Autodesk Inventor part; units mm, degrees
ref_plane "YZ Plane" through (0, 0, 0) normal (1, 0, 0) x (0, 1, 0)
ref_plane "XZ Plane" through (0, 0, 0) normal (0, 1, 0) x (-1, 0, 0)
ref_plane "XY Plane" through (0, 0, 0) normal (0, 0, 1) x (1, 0, 0)
sketch "Esquisse1" plane through (0, 0, 0) normal (0, 1, 0) x (-1, 0, 0)
  line L0 (60, -42) -> (60, 42)
  line L1 (55, 39) -> (57, 39)
  arc A0 (52, 42) -> (55, 39) centre (55, 42) ccw
  line L2 (52, 44) -> (52, 42)
  line L3 (55, 46) -> (-55, 46)
  circle A1 centre (55, 42.115) radius 2
  arc A2 (60, 42) -> (55, 47) centre (55, 42) ccw
  line L4 (55, 47) -> (-55, 47)
  line L5 (-55, 47) -> (55, 47)
  line L6 (51, 45) -> (-51, 45)
  line L7 (-52, 42) -> (-51, 42)
  arc A3 (-57, 39) -> (-58, 38) centre (-57, 38) ccw
  circle A4 centre (-55, 42.115) radius 2
  line L8 (-55, 39) -> (-55, 38)
  line L9 (-52, 44) -> (-52, 42)
  arc A5 (-51, 45) -> (-52, 44) centre (-51, 44) ccw
  line L10 (-55, 39) -> (-57, 39)
  arc A6 (-55, 39) -> (-52, 42) centre (-55, 42) ccw
  arc A7 (-57, 39) -> (-58, 38) centre (-57, 38) ccw
  circle A8 centre (55, -42.115) radius 2
  line L11 (-55, -39) -> (-57, -39)
  arc A9 (-52, -42) -> (-55, -39) centre (-55, -42) ccw
  line L12 (-52, -44) -> (-52, -42)
  line L13 (52, -42) -> (52, -44)
  circle A10 centre (-55, -42.115) radius 2
  line L14 (-51, -45) -> (51, -45)
  line L15 (51, -45) -> (-51, -45)
  line L16 (-55, -46) -> (55, -46)
  line L17 (-55, -47) -> (55, -47)
  line L18 (55, -47) -> (-55, -47)
  arc A11 (-51, 45) -> (-52, 44) centre (-51, 44) ccw
  line L19 (-52, 42) -> (-52, 44)
  arc A12 (-55, 46) -> (-59, 42) centre (-55, 42) ccw
  line L20 (-51, 42) -> (-51, 45)
  arc A13 (-55, 47) -> (-60, 42) centre (-55, 42) ccw
  circle A14 centre (-55, 42.115) radius 2
  line L21 (-55, 46) -> (-55, 47)
  arc A15 (-55, 47) -> (-60, 42) centre (-55, 42) ccw
  line L22 (52, -42) -> (51, -42)
  arc A16 (51, -45) -> (52, -44) centre (51, -44) ccw
  line L23 (-51, 45) -> (51, 45)
  arc A17 (52, 42) -> (55, 39) centre (55, 42) ccw
  line L24 (55, -39) -> (55, -38)
  line L25 (57, -39) -> (55, -39)
  line L26 (55, -39) -> (57, -39)
  arc A18 (55, -39) -> (52, -42) centre (55, -42) ccw
  arc A19 (57, -39) -> (58, -38) centre (57, -38) ccw
  line L27 (52, -44) -> (52, -42)
  arc A20 (51, -45) -> (52, -44) centre (51, -44) ccw
  circle A21 centre (55, -42.115) radius 2
  arc A22 (57, -39) -> (58, -38) centre (57, -38) ccw
  line L28 (58, 38) -> (58, -38)
  circle A23 centre (55, 42.115) radius 2
  line L29 (52, 42) -> (52, 44)
  line L30 (52, 42) -> (51, 42)
  arc A24 (52, 44) -> (51, 45) centre (51, 44) ccw
  line L31 (55, 39) -> (55, 38)
  arc A25 (52, 44) -> (51, 45) centre (51, 44) ccw
  arc A26 (58, 38) -> (57, 39) centre (57, 38) ccw
  arc A27 (58, 38) -> (57, 39) centre (57, 38) ccw
  line L32 (57, 39) -> (55, 39)
  line L33 (58, -38) -> (58, 38)
  line L34 (58, -38) -> (55, -38)
  line L35 (55, 46) -> (55, 47)
  arc A28 (59, 42) -> (55, 46) centre (55, 42) ccw
  arc A29 (60, 42) -> (55, 47) centre (55, 42) ccw
  line L36 (59, -42) -> (59, 42)
  line L37 (59, 42) -> (60, 42)
  line L38 (60, 42) -> (60, -42)
  line L39 (51, 45) -> (51, 42)
  arc A30 (51, 42) -> (55, 38) centre (55, 42) ccw
  line L40 (55, 38) -> (58, 38)
  arc A31 (55, -39) -> (52, -42) centre (55, -42) ccw
  arc A32 (55, -47) -> (60, -42) centre (55, -42) ccw
  line L41 (-55, -38) -> (-58, -38)
  arc A33 (-51, -42) -> (-55, -38) centre (-55, -42) ccw
  line L42 (-52, -42) -> (-51, -42)
  line L43 (-52, -42) -> (-52, -44)
  line L44 (-51, -45) -> (-51, -42)
  arc A34 (-52, -44) -> (-51, -45) centre (-51, -44) ccw
  circle A35 centre (-55, -42.115) radius 2
  line L45 (-55, -46) -> (-55, -47)
  arc A36 (-59, -42) -> (-55, -46) centre (-55, -42) ccw
  arc A37 (-60, -42) -> (-55, -47) centre (-55, -42) ccw
  line L46 (-60, -42) -> (-59, -42)
  arc A38 (-60, -42) -> (-55, -47) centre (-55, -42) ccw
  arc A39 (-58, -38) -> (-57, -39) centre (-57, -38) ccw
  line L47 (-57, 39) -> (-55, 39)
  arc A40 (-55, 39) -> (-52, 42) centre (-55, 42) ccw
  line L48 (-55, -39) -> (-55, -38)
  line L49 (-58, -38) -> (-58, 38)
  arc A41 (-52, -44) -> (-51, -45) centre (-51, -44) ccw
  arc A42 (-58, -38) -> (-57, -39) centre (-57, -38) ccw
  line L50 (-60, 42) -> (-60, -42)
  arc A43 (-52, -42) -> (-55, -39) centre (-55, -42) ccw
  line L51 (-57, -39) -> (-55, -39)
  line L52 (-58, 38) -> (-58, -38)
  line L53 (-58, 38) -> (-55, 38)
  arc A44 (-55, 38) -> (-51, 42) centre (-55, 42) ccw
  line L54 (-59, 42) -> (-60, 42)
  line L55 (-60, -42) -> (-60, 42)
  line L56 (-59, 42) -> (-59, -42)
  line L57 (55, -46) -> (55, -47)
  arc A45 (55, -38) -> (51, -42) centre (55, -42) ccw
  line L58 (51, -42) -> (51, -45)
  arc A46 (55, -46) -> (59, -42) centre (55, -42) ccw
  line L59 (59, -42) -> (60, -42)
  arc A47 (55, -47) -> (60, -42) centre (55, -42) ccw
  line L60 (-37.5, -35) -> (-22.5, -35)
  line L61 (-37.5, -35) -> (-22.5, -35)
  line L62 (-33.25, 35) -> (-37.5, 35)
  line L63 (-33.25, 35) -> (-31.25, 35)
  line L64 (-31.25, 32) -> (-33.25, 32)
  line L65 (-31.25, 35) -> (-31.25, 32)
  line L66 (-31.25, 32) -> (-33.25, 32)
  line L67 (-28.75, 35) -> (-31.25, 35)
  line L68 (-28.75, 32) -> (-28.75, 35)
  line L69 (-28.75, 32) -> (-28.75, 35)
  line L70 (-26.75, 32) -> (-28.75, 32)
  line L71 (-26.75, 32) -> (-28.75, 32)
  line L72 (-22.5, 35) -> (-37.5, 35)
  line L73 (-22.5, 35) -> (-26.75, 35)
  line L74 (-37.5, 35) -> (-37.5, -35)
  line L75 (-37.5, 35) -> (-37.5, -35)
  line L76 (-22.5, -35) -> (-22.5, 35)
  line L77 (-22.5, -35) -> (-22.5, 35)
  line L78 (-28.75, 35) -> (-26.75, 35)
  line L79 (-31.25, 35) -> (-31.25, 32)
  line L80 (-26.75, 35) -> (-26.75, 32)
  line L81 (-26.75, 35) -> (-26.75, 32)
  line L82 (-33.25, 32) -> (-33.25, 35)
  line L83 (-33.25, 32) -> (-33.25, 35)
  line L84 (-7.5, -35) -> (7.5, -35)
  line L85 (-7.5, -35) -> (7.5, -35)
  line L86 (-3.25, 35) -> (-7.5, 35)
  line L87 (-3.25, 35) -> (-1.25, 35)
  line L88 (-1.25, 32) -> (-3.25, 32)
  line L89 (-1.25, 35) -> (-1.25, 32)
  line L90 (-1.25, 32) -> (-3.25, 32)
  line L91 (1.25, 35) -> (-1.25, 35)
  line L92 (1.25, 32) -> (1.25, 35)
  line L93 (1.25, 32) -> (1.25, 35)
  line L94 (3.25, 32) -> (1.25, 32)
  line L95 (3.25, 32) -> (1.25, 32)
  line L96 (7.5, 35) -> (-7.5, 35)
  line L97 (7.5, 35) -> (3.25, 35)
  line L98 (-7.5, 35) -> (-7.5, -35)
  line L99 (-7.5, 35) -> (-7.5, -35)
  line L100 (7.5, -35) -> (7.5, 35)
  line L101 (7.5, -35) -> (7.5, 35)
  line L102 (1.25, 35) -> (3.25, 35)
  line L103 (-1.25, 35) -> (-1.25, 32)
  line L104 (3.25, 35) -> (3.25, 32)
  line L105 (3.25, 35) -> (3.25, 32)
  line L106 (-3.25, 32) -> (-3.25, 35)
  line L107 (-3.25, 32) -> (-3.25, 35)
  line L108 (22.5, -35) -> (37.5, -35)
  line L109 (22.5, -35) -> (37.5, -35)
  line L110 (26.75, 35) -> (22.5, 35)
  line L111 (26.75, 35) -> (28.75, 35)
  line L112 (28.75, 32) -> (26.75, 32)
  line L113 (28.75, 35) -> (28.75, 32)
  line L114 (28.75, 32) -> (26.75, 32)
  line L115 (31.25, 35) -> (28.75, 35)
  line L116 (31.25, 32) -> (31.25, 35)
  line L117 (31.25, 32) -> (31.25, 35)
  line L118 (33.25, 32) -> (31.25, 32)
  line L119 (33.25, 32) -> (31.25, 32)
  line L120 (37.5, 35) -> (22.5, 35)
  line L121 (37.5, 35) -> (33.25, 35)
  line L122 (22.5, 35) -> (22.5, -35)
  line L123 (22.5, 35) -> (22.5, -35)
  line L124 (37.5, -35) -> (37.5, 35)
  line L125 (37.5, -35) -> (37.5, 35)
  line L126 (31.25, 35) -> (33.25, 35)
  line L127 (28.75, 35) -> (28.75, 32)
  line L128 (33.25, 35) -> (33.25, 32)
  line L129 (33.25, 35) -> (33.25, 32)
  line L130 (26.75, 32) -> (26.75, 35)
  line L131 (26.75, 32) -> (26.75, 35)
  line L132 (55, -42) -> (-55, 42) construction
  line L133 (55, 42) -> (-55, -42) construction
  line L134 (58, -30.8976) -> (-58, -30.8976)
  point P0 (0, 0)
  point P1 (0, 0)
  point P2 (37.5, -30.8976)
  point P3 (22.5, -30.8976)
  point P4 (7.5, -30.8976)
  point P5 (-7.5, -30.8976)
  point P6 (-22.5, -30.8976)
  point P7 (-37.5, -30.8976)
  point P8 (-58, -30.8976)
extrude "Extrusion1" add sketch "Esquisse1" along normal blind 5 contours L28 L34 A45 L58 L14 L44 A33 L41 L49 L134 L74 L60 L76 L98 L84 L100 L122 L108 L124
sketch "Esquisse2" plane through (0, 5, 0) normal (0, 1, 0) x (1, 0, 0)
  line L0 (-58, 38) -> (-58, 30.8976)
  line L1 (-58, 30.8976) -> (-37.5, 30.8976)
  line L2 (-37.5, 30.8976) -> (-37.5, 35)
  line L3 (-37.5, 35) -> (-22.5, 35)
  line L4 (-22.5, 35) -> (-22.5, 30.8976)
  line L5 (-22.5, 30.8976) -> (-7.5, 30.8976)
  line L6 (-7.5, 30.8976) -> (-7.5, 35)
  line L7 (-7.5, 35) -> (7.5, 35)
  line L8 (7.5, 35) -> (7.5, 30.8976)
  line L9 (7.5, 30.8976) -> (22.5, 30.8976)
  line L10 (22.5, 30.8976) -> (22.5, 35)
  line L11 (22.5, 35) -> (37.5, 35)
  line L12 (37.5, 35) -> (37.5, 30.8976)
  line L13 (37.5, 30.8976) -> (58, 30.8976)
  line L14 (58, 30.8976) -> (58, 38)
  line L15 (58, 38) -> (55, 38)
  arc A0 (51, 42) -> (55, 38) centre (55, 42) ccw
  line L16 (51, 42) -> (51, 45)
  line L17 (51, 45) -> (-51, 45)
  line L18 (-51, 45) -> (-51, 42)
  arc A1 (-55, 38) -> (-51, 42) centre (-55, 42) ccw
  line L19 (-55, 38) -> (-58, 38)
  line L20 (-50.9, 44.9) -> (50.9, 44.9)
  line L21 (50.9, 44.9) -> (50.9, 42)
  arc A2 (50.9, 42) -> (55, 37.9) centre (55, 42) ccw
  line L22 (55, 37.9) -> (57.9, 37.9)
  line L23 (57.9, 37.9) -> (57.9, 30.9976)
  line L24 (57.9, 30.9976) -> (37.6, 30.9976)
  line L25 (37.6, 30.9976) -> (37.6, 35.1)
  line L26 (37.6, 35.1) -> (22.4, 35.1)
  line L27 (22.4, 35.1) -> (22.4, 30.9976)
  line L28 (22.4, 30.9976) -> (7.6, 30.9976)
  line L29 (7.6, 30.9976) -> (7.6, 35.1)
  line L30 (7.6, 35.1) -> (-7.6, 35.1)
  line L31 (-7.6, 35.1) -> (-7.6, 30.9976)
  line L32 (-7.6, 30.9976) -> (-22.4, 30.9976)
  line L33 (-22.4, 30.9976) -> (-22.4, 35.1)
  line L34 (-22.4, 35.1) -> (-37.6, 35.1)
  line L35 (-37.6, 35.1) -> (-37.6, 30.9976)
  line L36 (-37.6, 30.9976) -> (-57.9, 30.9976)
  line L37 (-57.9, 30.9976) -> (-57.9, 37.9)
  line L38 (-57.9, 37.9) -> (-55, 37.9)
  arc A3 (-55, 37.9) -> (-50.9, 42) centre (-55, 42) ccw
  line L39 (-50.9, 42) -> (-50.9, 44.9)
  point P0 (0, 0)
  dimension "d2" = 0.1
extrude "Extrusion2" cut sketch "Esquisse2" against normal blind 5
chamfer "Chanfrein1" distance 3 angle 45 3 edges at (-30, 5, -35.1) (0, 5, -35.1) (30, 5, -35.1)
fillet "Congé1" radius 1 6 edges at (-37.6, 2.5, -30.9976) (-22.4, 2.5, -30.9976) (-7.6, 2.5, -30.9976) (7.6, 2.5, -30.9976) (22.4, 2.5, -30.9976) (37.6, 2.5, -30.9976)
sketch "Esquisse4" plane through (0, 5, 0) normal (0, 1, 0) x (1, 0, 0)
  line L0 (-33.3, 31.1) -> (-26.7, 31.1)
  line L1 (-26.7, 31.1) -> (-26.7, 39.1)
  line L2 (-26.7, 39.1) -> (-33.3, 39.1)
  line L3 (-33.3, 39.1) -> (-33.3, 31.1)
  line L4 (-22.4, 35.1) -> (-37.6, 35.1)
  line L5 (-33.3, 31.1) -> (-26.7, 39.1) construction
  line L6 (-26.7, 31.1) -> (-33.3, 39.1) construction
  line L7 (-3.3, 31.1) -> (3.3, 31.1)
  line L8 (3.3, 31.1) -> (3.3, 39.1)
  line L9 (3.3, 39.1) -> (-3.3, 39.1)
  line L10 (-3.3, 39.1) -> (-3.3, 31.1)
  line L11 (7.6, 35.1) -> (-7.6, 35.1)
  line L12 (-3.3, 31.1) -> (3.3, 39.1) construction
  line L13 (3.3, 31.1) -> (-3.3, 39.1) construction
  line L14 (26.7, 31.1) -> (33.3, 31.1)
  line L15 (33.3, 31.1) -> (33.3, 39.1)
  line L16 (33.3, 39.1) -> (26.7, 39.1)
  line L17 (26.7, 39.1) -> (26.7, 31.1)
  line L18 (37.6, 35.1) -> (22.4, 35.1)
  line L19 (26.7, 31.1) -> (33.3, 39.1) construction
  line L20 (33.3, 31.1) -> (26.7, 39.1) construction
  point P0 (0, 0)
  point P1 (-30, 35.1)
  point P2 (0, 35.1)
  point P3 (30, 35.1)
  point P4 (26.7, 35.1)
  point P5 (33.3, 35.1)
  point P6 (-3.3, 35.1)
  point P7 (3.3, 35.1)
  point P8 (-33.3, 35.1)
  point P9 (-26.7, 35.1)
  dimension "d9" = 6.6
  dimension "d10" = 8
  dimension "d11" = 6.6
  dimension "d12" = 8
  dimension "d13" = 6.6
extrude "Extrusion3" cut sketch "Esquisse4" against normal blind 5 contours L3 L2 L1 L4 | L10 L9 L8 L11 | L17 L16 L15 L18
chamfer "Chanfrein2" distance 3 angle 45 3 edges at (-30, 5, -39.1) (0, 5, -39.1) (30, 5, -39.1)
properties part number "Centreur_resistance"
Check sheet for the modelled part. Datum: model origin and axes. Units: mm. A direction names the side the tool comes from. Round coordinates to 2 decimals unless told otherwise and drop trailing zeros. Write each loop counter-clockwise with the first axis right and the second up, starting at its lowest first coordinate (ties: lowest second). Pieces come first, ordered by that corner, then holes. Notation, with made-up numbers: (58.5, -25) - (100.5, -25) arc R18 ccw to (100.5, -6) - close; hole circle Ø3 at (13, 89). An arc over 180 degrees is marked (long way). Return JSON: item names as keys, results as strings.
Q1. Access from +Z, -Z, +X, -X, +Y, -Y to the whole of each face (thin tool, end or side, straight path). Record for faces 1 (the flat face through (-48, 3, -30.998)), 2 (the flat face through (-5, 1, -35.1)), 3 (the flat face through (-7.6, 3, -34)), 4 (the flat face through (50.9, 3, -43)).
Returned:
{"face 1": "+Z, +X, -X, +Y, -Y", "face 2": "+Z, +Y, -Y", "face 3": "+Z, +Y", "face 4": "-Z, +X, +Y, -Y"}
Q2. Cross-section at B-B (x = 29). Record the boundary of the cut face in (y, z).
Returned:
{"outline": "(0, -44.9) - (5, -44.9) - (5, -42.1) - (2, -39.1) - (0, -39.1) - close"}
Q3. Draft check along X on faces 5 (the flat face through (0, 1, -39.1)), 6 (the flat face through (48, 3, -30.998)), 7 (the flat face through (-22.4, 3, -34)), 8 (the flat face through (-50.9, 3, -43)). Enter one of: released by +X, released by -X, zero draft, split by the parting line, or undercut.
Returned:
{"face 5": "undercut", "face 6": "zero draft", "face 7": "undercut", "face 8": "released by -X"}
Q4. Cross-section at A-A (z = -34). Record the boundary of the cut face in (x, y), then the cut area to 3 significant figures.
Returned:
{"outline": "(-57.9, 0) - (-37.6, 0) - (-37.6, 5) - (-57.9, 5) - close; (-22.4, 0) - (-7.6, 0) - (-7.6, 5) - (-22.4, 5) - close; (7.6, 0) - (22.4, 0) - (22.4, 5) - (7.6, 5) - close; (37.6, 0) - (57.9, 0) - (57.9, 5) - (37.6, 5) - close", "area": "351 mm²"}
Q5. Scan lines: L1, parallel to X at y = 2.6, z = -37.75; L2, parallel to X at y = 0.85, z = -34; L3, parallel to Z at x = -7.5, y = 1.1. Record each from-to range of solid material in increasing order. Write a range as from..to.
Returned:
{"L1": "x = -57.9..-33.3, -26.7..-3.3, 3.3..26.7, 33.3..57.9", "L2": "x = -57.9..-37.6, -22.4..-7.6, 7.6..22.4, 37.6..57.9", "L3": "z = -44.9..-35.1"}
Q6. Depth check by flat-ended pin: P1, Ø2, axis at y = 3.5, z = -41, coming from the -X side; P2, Ø2, axis at x = 30.5, y = 1, coming from the +Z side; P3, Ø3, axis at y = 3, z = -43.5, coming from the -X side; P4, Ø5, axis at x = -39.5, z = -38, coming from the -Y side. Enter the tip coordinate at first touch or a pass-through.
Returned:
{"P1": "stops at x = -51.42", "P2": "stops at z = -39.1", "P3": "stops at x = -50.9", "P4": "stops at y = 0"}
